```python
from build123d import *

# Parameters (mm, degrees)
EXTRUDE_1_DEPTH = 700


with BuildPart() as part:
    # 草图1 → 凸台-拉伸1 (new body)
    with BuildSketch(Plane.XY):
        with BuildLine():
            ThreePointArc((167.391004131, -248.958333333), (212.132034356, -212.132034356), (248.958333333, -167.391004131))
            ThreePointArc((248.958333333, -167.391004131), (475, 0), (248.958333333, 167.391004131))
            ThreePointArc((248.958333333, 167.391004131), (212.132034356, 212.132034356), (167.391004131, 248.958333333))
            ThreePointArc((167.391004131, 248.958333333), (0, 475), (-167.391004131, 248.958333333))
            ThreePointArc((-167.391004131, 248.958333333), (-212.132034356, 212.132034356), (-248.958333333, 167.391004131))
            ThreePointArc((-248.958333333, 167.391004131), (-475, 0), (-248.958333333, -167.391004131))
            ThreePointArc((-248.958333333, -167.391004131), (-212.132034356, -212.132034356), (-167.391004131, -248.958333333))
            ThreePointArc((-167.391004131, -248.958333333), (0, -475), (167.391004131, -248.958333333))
        make_face()
    extrude(amount=EXTRUDE_1_DEPTH)

    # 草图2 → 切除-旋转1 (revolve, cut)
    with BuildSketch(Plane(origin=(0, 0, 0), x_dir=(1, 0, 0), z_dir=(0, 1, 0)), mode=Mode.PRIVATE) as cut_revolve_1_sk:
        Polygon((500, -400), (500, 0), (300, 0), (300, -300), align=None)
    revolve(cut_revolve_1_sk.sketch.rotate(Axis((0, 0, 700), (0, 0, -1)), 146.0844734), axis=Axis((0, 0, 700), (0, 0, -1)), mode=Mode.SUBTRACT)


solid = part.part
```
Build history of the part. All positions in model axes, mm. Coordinates: 2 decimals unless noted, no trailing zeros. Order: outer loops, then holes, each group sorted by start corner. A loop starts at its lowest first (then second) coordinate and runs counter-clockwise, first axis right, second up. Notation, with made-up numbers: (84.5, 9.25) -> (104.5, 9.25) arc R15 cw to (104.5, 31.25) -> close; hole circle Ø8 at (-32.5, 2). An arc over 180 degrees is marked (long way). Answer in a Markdown table with one row per item. Add a question column.
Q1. Mould opens along X. For faces 1 (the face through (-7, 7, 700)), 2 (the face through (474.94, -4.57, 541.64)), 3 (the face through (-4.57, -474.94, 541.64)) say: +X half, -X half, draft (parallel to the pull), parting line (faces both ways), or undercut.
Q2. Band-saw the part on A-A, the plane x = 0. List the corners of the cut face in (y, z).
Q3. Band-saw the part on C-C, the plane y = 231. List the corners of the cut face in (x, z), then the cut area to 3 significant figures.
Q4. Band-saw the part on B-B, the plane z = 640. List the corners of the cut face in (x, y).
Q5. Band-saw the part on D-D, the plane y = -191.5. List the corners of the cut face in (x, z), then the cut area to 3 significant figures.
Q6. Wall check: line 1 along X through (y, z) = (-306, 475); line 2 along X through (y, z) = (249.5, 544.5); line 3 along Y through (x, z) = (-372, 410). Give the ranges that are in metal, low to high. Write a range as [from, to].
Q7. Drop flat-ended pins along their axis: pin 1 (4 mm diameter, centred on y = -211, z = 469, fed in from -X); pin 2 (5 mm diameter, centred on y = 173, z = 210.5, fed in from +X); pin 3 (12 mm diameter, centred on y = -202, z = 186, fed in from +X). Give the stop position or say it passes through.
Answers follow:
| question | item | result |
|---|---|---|
| 1 | face 1 | draft |
| 1 | face 2 | undercut |
| 1 | face 3 | parting line |
| 2 | outline | (-475, 387.5) -> (-300, 300) -> (-300, 0) -> (300, 0) -> (300, 300) -> (475, 387.5) -> (475, 700) -> (-475, 700) -> close |
| 3 | outline | (-191.41, 0) -> (191.41, 0) -> (191.41, 700) -> (-191.41, 700) -> close |
| 3 | area | 268,000 mm^2 |
| 4 | outline | (-248.96, -167.39) arc R300 ccw to (-167.39, -248.96) arc R175 ccw (long way) to (167.39, -248.96) arc R300 ccw to (248.96, -167.39) arc R175 ccw (long way) to (248.96, 167.39) arc R300 ccw to (167.39, 248.96) arc R175 ccw (long way) to (-167.39, 248.96) arc R300 ccw to (-248.96, 167.39) arc R175 ccw (long way) to start |
| 5 | outline | (-230.93, 0) -> (230.93, 0) -> (230.93, 700) -> (-230.93, 700) -> close |
| 5 | area | 323,000 mm^2 |
| 6 | line 1 | [-174.9, 174.9] |
| 6 | line 2 | [-167.56, 167.56] |
| 6 | line 3 | [-159.5, 159.5] |
| 7 | pin 1 | x = -215.22 |
| 7 | pin 2 | x = 246.84 |
| 7 | pin 3 | x = 227.12 |
